Can you work these out from the model? Positions are in its coordinate system, mm. A direction names the side the tool comes from. Round coordinates to 2 decimals unless told otherwise and drop trailing zeros. Loops run counter-clockwise (first coordinate to the right, second up) from the corner with the lowest first, then second, coordinate; pieces in that order, holes last.
```python
from build123d import *

# Parameters (mm, degrees)
SKETCH1_R             = 40
SKETCH1_R_2           = 16
BOSS_EXTRUDE2_DEPTH   = 10
SKETCH1_R_3           = 20
SKETCH1_R_4           = 15
BOSS_EXTRUDE2_2_DEPTH = 10
BOSS_EXTRUDE2_3_DEPTH = 10
SKETCH1_4_R           = 15
BOSS_EXTRUDE3_DEPTH   = 7.5


with BuildPart() as part:
    # Sketch1 → Boss-Extrude2 (new, symmetric)
    with BuildSketch(Plane.XY):
        Circle(SKETCH1_R)
        Circle(SKETCH1_R_2, mode=Mode.SUBTRACT)
        with BuildLine():
            Line((-3, -20.784609691), (-3, -31.859064644))
            ThreePointArc((-3, -31.859064644), (-16, -27.712812921), (-26.090759323, -18.527608533))
            Line((-26.090759323, -18.527608533), (-16.5, -12.990381057))
            ThreePointArc((-16.5, -12.990381057), (-10.5, -18.186533479), (-3, -20.784609691))
        make_face(mode=Mode.SUBTRACT)
        with BuildLine():
            Line((3, -20.784609691), (3, -31.859064644))
            ThreePointArc((3, -31.859064644), (16, -27.712812921), (26.090759323, -18.527608533))
            Line((26.090759323, -18.527608533), (16.5, -12.990381057))
            ThreePointArc((16.5, -12.990381057), (10.5, -18.186533479), (3, -20.784609691))
        make_face(mode=Mode.SUBTRACT)
        with BuildLine():
            Line((-19.5, -7.794228634), (-29.090759323, -13.331456111))
            ThreePointArc((-29.090759323, -13.331456111), (-32, 0), (-29.090759323, 13.331456111))
            Line((-29.090759323, 13.331456111), (-19.5, 7.794228634))
            ThreePointArc((-19.5, 7.794228634), (-21, 0), (-19.5, -7.794228634))
        make_face(mode=Mode.SUBTRACT)
        with BuildLine():
            Line((-16.5, 12.990381057), (-26.090759323, 18.527608533))
            ThreePointArc((-26.090759323, 18.527608533), (-16, 27.712812921), (-3, 31.859064644))
            Line((-3, 31.859064644), (-3, 20.784609691))
            ThreePointArc((-3, 20.784609691), (-10.5, 18.186533479), (-16.5, 12.990381057))
        make_face(mode=Mode.SUBTRACT)
        with BuildLine():
            Line((3, 20.784609691), (3, 31.859064644))
            ThreePointArc((3, 31.859064644), (16, 27.712812921), (26.090759323, 18.527608533))
            Line((26.090759323, 18.527608533), (16.5, 12.990381057))
            ThreePointArc((16.5, 12.990381057), (10.5, 18.186533479), (3, 20.784609691))
        make_face(mode=Mode.SUBTRACT)
        with BuildLine():
            Line((19.5, 7.794228634), (29.090759323, 13.331456111))
            ThreePointArc((29.090759323, 13.331456111), (32, 0), (29.090759323, -13.331456111))
            Line((29.090759323, -13.331456111), (19.5, -7.794228634))
            ThreePointArc((19.5, -7.794228634), (21, 0), (19.5, 7.794228634))
        make_face(mode=Mode.SUBTRACT)
    extrude(amount=BOSS_EXTRUDE2_DEPTH, both=True)



with BuildPart() as body_2:
    # Sketch1 → Boss-Extrude2 2 (new, symmetric)
    with BuildSketch(Plane.XY):
        with Locations((70, 0)):
            Circle(SKETCH1_R_3)
        with Locations((70, 0)):
            Circle(SKETCH1_R_4, mode=Mode.SUBTRACT)
    extrude(amount=BOSS_EXTRUDE2_2_DEPTH, both=True)


with BuildPart() as body_3:
    # Sketch1 → Boss-Extrude2 3 (new, symmetric)
    with BuildSketch(Plane.XY):
        with Locations(Location((-70, 0, 0), (0, 0, 180))):
            Circle(SKETCH1_R_3)
        with Locations(Location((-70, 0, 0), (0, 0, 180))):
            Circle(SKETCH1_R_4, mode=Mode.SUBTRACT)
    extrude(amount=BOSS_EXTRUDE2_3_DEPTH, both=True)


with BuildPart() as part_1:
    add(part.part)

    add(body_2.part)  # Boss-Extrude3 merges body 2

    add(body_3.part)  # Boss-Extrude3 merges body 3
    # Sketch1_4 → Boss-Extrude3 (add, symmetric)
    # profile 1 of 2: a face of its own
    with BuildSketch(Plane.XY):
        with BuildLine():
            Line((89.071294105, 6.023764702), (70.02485881, 66.324952937))
            ThreePointArc((70.02485881, 66.324952937), (46.6282273, 80.727545655), (29.002885891, 59.651863383))
            ThreePointArc((29.002885891, 59.651863383), (22.168588856, 44.262528341), (6.003756239, 39.546869801))
            ThreePointArc((6.003756239, 39.546869801), (30.332740146, 26.075369129), (40, 0))
            ThreePointArc((40, 0), (30.332740146, -26.075369129), (6.003756239, -39.546869801))
            ThreePointArc((6.003756239, -39.546869801), (22.168588856, -44.262528341), (29.002885891, -59.651863383))
            ThreePointArc((29.002885891, -59.651863383), (46.6282273, -80.727545655), (70.02485881, -66.324952937))
            Line((70.02485881, -66.324952937), (89.071294105, -6.023764702))
            ThreePointArc((89.071294105, -6.023764702), (50, 0), (89.071294105, 6.023764702))
        make_face()
        with Locations((50, -60)):
            Circle(SKETCH1_4_R, mode=Mode.SUBTRACT)
        with Locations((50, 60)):
            Circle(SKETCH1_4_R, mode=Mode.SUBTRACT)
    # profile 2 of 2: a face of its own
    with BuildSketch(Plane.XY):
        with BuildLine():
            ThreePointArc((-6.003756239, -39.546869801), (-40, 0), (-6.003756239, 39.546869801))
            ThreePointArc((-6.003756239, 39.546869801), (-22.168588856, 44.262528341), (-29.002885891, 59.651863383))
            ThreePointArc((-29.002885891, 59.651863383), (-46.6282273, 80.727545655), (-70.02485881, 66.324952937))
            Line((-70.02485881, 66.324952937), (-89.071294105, 6.023764702))
            ThreePointArc((-89.071294105, 6.023764702), (-66.95253237, 19.766460003), (-50, 0))
            ThreePointArc((-50, 0), (-66.95253237, -19.766460003), (-89.071294105, -6.023764702))
            Line((-89.071294105, -6.023764702), (-70.02485881, -66.324952937))
            ThreePointArc((-70.02485881, -66.324952937), (-46.6282273, -80.727545655), (-29.002885891, -59.651863383))
            ThreePointArc((-29.002885891, -59.651863383), (-22.168588856, -44.262528341), (-6.003756239, -39.546869801))
        make_face()
        with Locations((-50, -60)):
            Circle(SKETCH1_4_R, mode=Mode.SUBTRACT)
        with Locations((-50, 60)):
            Circle(SKETCH1_4_R, mode=Mode.SUBTRACT)
    extrude(amount=BOSS_EXTRUDE3_DEPTH, both=True)


solid = part_1.part
```
(1) We'd pull the mould along X, two halves only. Please class faces 4 (the flat face through (73, 15, 10)), 5 (the cylindrical face through (-62, 51, 0)): released by +X, released by -X, zero draft, split by the parting line, or undercut.
(2) Suppose I cut it at D-D (x = -45.5). Write out the boundary of the cut face in (y, z).
(3) Suppose I cut it at C-C (y = 55.5). Write out the boundary of the cut face in (x, z), then the cut area to 3 significant figures.
(4) For pin 1 (25 mm diameter, centred on x = 45.5, y = -32.5, fed in from -Z); pin 2 (24 mm diameter, centred on x = -50, y = 60, fed in from +Z); pin 3 (3.5 mm diameter, centred on y = -29, z = 0.5, fed in from +X); pin 4 (1 mm diameter, centred on x = -20.5, z = -2.5, fed in from +Y), each with a flat end and sliding along its axis, tell me the tip position at first contact or that it passes through.
(5) Which directions (+Z, -Z, +X, -X, +Y, -Y) give clear straight access to the entire face, cutting with the end or side of a thin tool? Please do faces 1 (the flat face through (3, -26, 0)), 2 (the flat face through (47, 6, -7.5)), 3 (the flat face through (47, 6, 7.5)).
(6) If I drill on line 1 (Y direction, x = -50, z = 2.75); line 2 (Y direction, x = 0, z = -4.75); line 3 (X direction, y = -26, z = -6.5), over which ranges is the centre line in solid material (lowest first)?
(7) Suppose I cut it at B-B (x = -73). Write out the boundary of the cut face in (y, z), then the cut area to 3 significant figures.
(8) Suppose I cut it at A-A (y = -29). Write out the boundary of the cut face in (x, z).
Check result:
1. face 4: zero draft
1. face 5: undercut
2. outline: (-80.51, -7.5) - (-74.31, -7.5) - (-74.31, 7.5) - (-80.51, 7.5) - close; (-45.69, -7.5) - (45.69, -7.5) - (45.69, 7.5) - (-45.69, 7.5) - close; (74.31, -7.5) - (80.51, -7.5) - (80.51, 7.5) - (74.31, 7.5) - close
3. outline: (-73.44, -7.5) - (-64.31, -7.5) - (-64.31, 7.5) - (-73.44, 7.5) - close; (-35.69, -7.5) - (-28.64, -7.5) - (-28.64, 7.5) - (-35.69, 7.5) - close; (28.64, -7.5) - (35.69, -7.5) - (35.69, 7.5) - (28.64, 7.5) - close; (64.31, -7.5) - (73.44, -7.5) - (73.44, 7.5) - (64.31, 7.5) - close
3. area: 486 mm2
4. pin 1: stops at z = -7.5
4. pin 2: passes through
4. pin 3: stops at x = 82.37
4. pin 4: stops at y = 43.32
5. face 1: +Z, -Z
5. face 2: -Z
5. face 3: +Z
6. line 1: y = -81 to -75, -45 to 45, 75 to 81
6. line 2: y = -40 to -16, 16 to 40
6. line 3: x = -82.76 to -18.65, -3 to 3, 18.65 to 82.76
7. outline: (-56.91, -7.5) - (-19.77, -7.5) - (-19.77, -10) - (-14.7, -10) - (-14.7, 10) - (-19.77, 10) - (-19.77, 7.5) - (-56.91, 7.5) - close; (14.7, -10) - (19.77, -10) - (19.77, -7.5) - (56.91, -7.5) - (56.91, 7.5) - (19.77, 7.5) - (19.77, 10) - (14.7, 10) - close
7. area: 1,320 mm2
8. outline: (-81.81, -7.5) - (-27.55, -7.5) - (-27.55, -10) - (-13.53, -10) - (-13.53, 10) - (-27.55, 10) - (-27.55, 7.5) - (-81.81, 7.5) - close; (-3, -10) - (3, -10) - (3, 10) - (-3, 10) - close; (13.53, -10) - (27.55, -10) - (27.55, -7.5) - (81.81, -7.5) - (81.81, 7.5) - (27.55, 7.5) - (27.55, 10) - (13.53, 10) - close
